Check sheet for the modelled part. Datum: model origin and axes. Units: mm. Face numbers are marked on the shaded views. Coordinates: 2 decimals unless noted, no trailing zeros. Loops run counter-clockwise (first coordinate to the right, second up) from the corner with the lowest first, then second, coordinate; pieces in that order, holes last.
from build123d import *

# Parameters (mm, degrees)
SKETCH1_W           = 89
SKETCH1_H           = 70
SKETCH1_R           = 1
BOSS_EXTRUDE1_DEPTH = 10
CUT_EXTRUDE2_DEPTH  = 7


with BuildPart() as part:
    # Sketch1 → Boss-Extrude1 (new body)
    with BuildSketch(Plane(origin=(0, 0, 0), x_dir=(1, 0, 0), z_dir=(0, 1, 0))):
        Rectangle(SKETCH1_W, SKETCH1_H)
        with Locations(Location((-39.5, 30, 0), (0, 0, 270))):
            Circle(SKETCH1_R, mode=Mode.SUBTRACT)
        with Locations(Location((39.5, 30, 0), (0, 0, 90))):
            Circle(SKETCH1_R, mode=Mode.SUBTRACT)
        with Locations(Location((39.5, -30, 0), (0, 0, 270))):
            Circle(SKETCH1_R, mode=Mode.SUBTRACT)
        with Locations(Location((-39.5, -30, 0), (0, 0, 90))):
            Circle(SKETCH1_R, mode=Mode.SUBTRACT)
    extrude(amount=BOSS_EXTRUDE1_DEPTH)

    # Sketch3 → Cut-Extrude2 (cut)
    with BuildSketch(Plane(origin=(0, 10, 0), x_dir=(1, 0, 0), z_dir=(0, 1, 0))):
        Polygon((-44.5, -20), (-29.5, -35), (29.5, -35), (44.5, -20), (44.5, 20), (29.5, 35), (-29.5, 35), (-44.5, 20), align=None)
    extrude(amount=-CUT_EXTRUDE2_DEPTH, mode=Mode.SUBTRACT)


solid = part.part
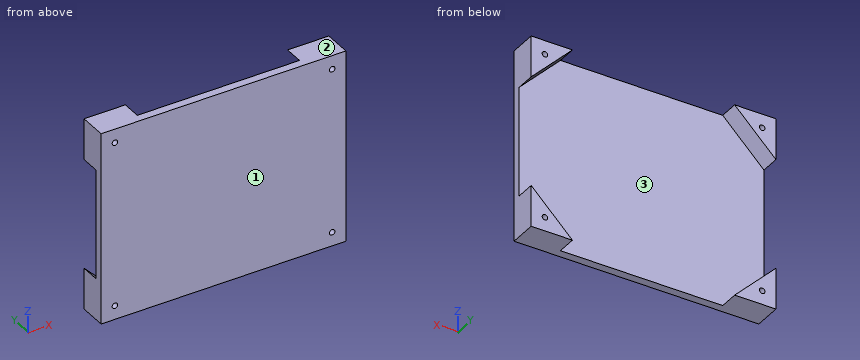
(1) Section check B-B, the plane x = 39.5. Enter the section's corners in (y, z), plus the area to 3 significant figures.
(2) Gauge pin test, flat ends, axial feed: P1, Ø5, axis at x = 16, z = -2.5, coming from the +Y side; P2, Ø6, axis at x = 8, y = 5, coming from the +Z side. Record the tip position at first contact, or that the pin passes through.
(3) Draft check along Z on the marked faces 1, 2 and 3. Enter one of: pulls with the +Z half, pulls with the -Z half, needs draft (parallel to the pull), parting line crosses it, or undercut.
(4) Section check A-A, the plane y = 6.5. Enter the section's corners in (x, z).
(5) Section check D-D, the plane z = -21. Enter the section's corners in (x, y), plus the area to 3 significant figures.
(6) Section check C-C, the plane z = 30. Enter the section's corners in (x, y).
(7) Scan lines: line 1 along X through (y, z) = (7.5, -30); line 2 along Y through (x, z) = (41.5, -5); line 3 along Z through (x, y) = (-40, 0.75). Record each from-to range of solid material in increasing order.
Determined:
1. outline: (0, -35) - (10, -35) - (10, -31) - (0, -31) - close; (0, -29) - (10, -29) - (10, -25) - (3, -25) - (3, 25) - (10, 25) - (10, 29) - (0, 29) - close; (0, 31) - (10, 31) - (10, 35) - (0, 35) - close
1. area: 310 mm2
2. P1: stops at y = 3
2. P2: stops at z = 35
3. face 1: needs draft
3. face 2: pulls with the +Z half
3. face 3: undercut
4. outline: (-44.5, -35) - (-29.5, -35) - (-44.5, -20) - close; (-44.5, 20) - (-29.5, 35) - (-44.5, 35) - close; (29.5, -35) - (44.5, -35) - (44.5, -20) - close; (29.5, 35) - (44.5, 20) - (44.5, 35) - close; hole circle Ø2 at (-39.5, -30); hole circle Ø2 at (-39.5, 30); hole circle Ø2 at (39.5, -30); hole circle Ø2 at (39.5, 30)
5. outline: (-44.5, 0) - (44.5, 0) - (44.5, 10) - (43.5, 10) - (43.5, 3) - (-43.5, 3) - (-43.5, 10) - (-44.5, 10) - close
5. area: 281 mm2
6. outline: (-44.5, 0) - (-40.5, 0) - (-40.5, 10) - (-44.5, 10) - close; (-38.5, 0) - (38.5, 0) - (38.5, 10) - (34.5, 10) - (34.5, 3) - (-34.5, 3) - (-34.5, 10) - (-38.5, 10) - close; (40.5, 0) - (44.5, 0) - (44.5, 10) - (40.5, 10) - close
7. line 1: x = -44.5 to -40.5, -38.5 to -34.5, 34.5 to 38.5, 40.5 to 44.5
7. line 2: y = 0 to 3
7. line 3: z = -35 to -30.87, -29.13 to 29.13, 30.87 to 35
